The drawing under review shows one solid part. Ordinate dimensions are in mm from its lowest x, y, z. A direction names the side the tool comes from. Give positions to 0.01 mm unless a question says otherwise; leave off trailing zeros. Order: outer loops, then holes, each group sorted by start corner. A loop starts at its lowest first (then second) coordinate and runs counter-clockwise, first axis right, second up. Notation, with made-up numbers: M 17,13 L 23,13 A20 ccw 23,41 Z; hole C 35.5,55 d9. An arc over 180 degrees is marked long. Put each result on its own line as item: value. Start each with the question number.
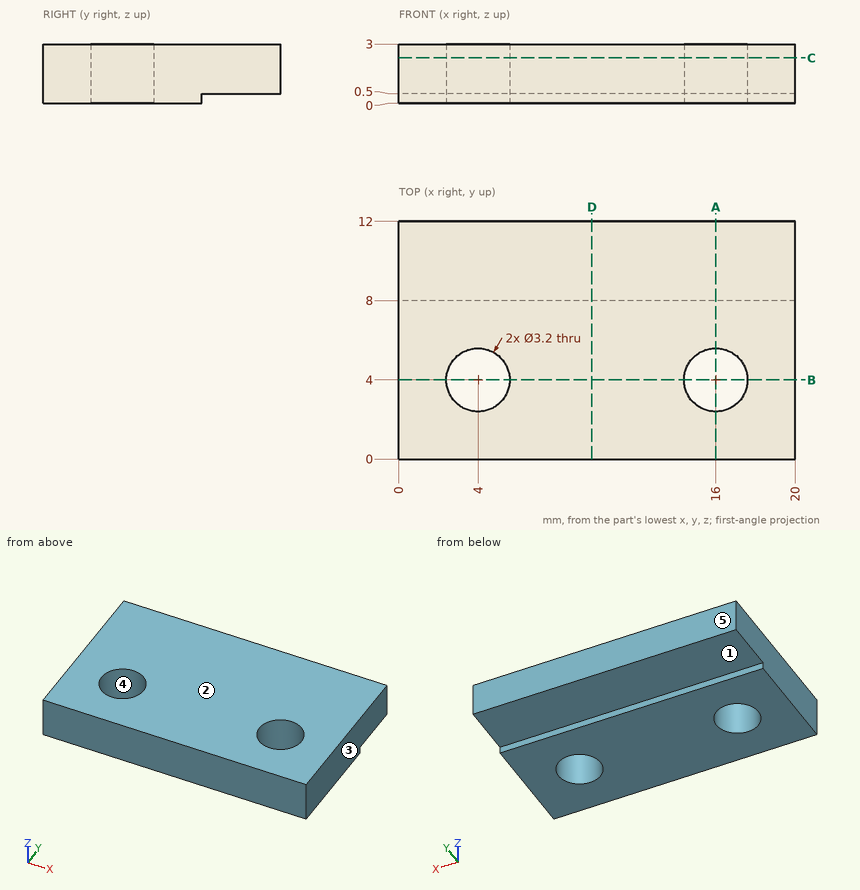
1. To check wall thickness, follow probe 1 along Y at (x, z) = (4, 1.35); probe 2 along X at (y, z) = (5.25, 1.4); probe 3 along Z at (x, y) = (18.75, 10.5). State the ranges of each line that lie inside material, in increasing order.
2. Consider section B-B on y = 4. Give the boundary of the cut face in (x, z), then the cut area to 3 significant figures.
3. Consider section C-C on z = 2.3. Give the boundary of the cut face in (x, y), then the cut area to 3 significant figures.
4. The part is to be moulded in two halves that separate along X. For the marked faces 3, 4 and 5, say which applies: +X half, -X half, draft (parallel to the pull), parting line (faces both ways), or undercut.
5. Insertion check: pin 1 (2 mm diameter, centred on x = 13, y = 10, fed in from -Z); pin 2 (3 mm diameter, centred on x = 4, y = 4, fed in from -Z). Each pin has a flat end and moves straight along its axis. Give the tip position at first contact, or say it passes through.
6. Consider section A-A on x = 16. Give the boundary of the cut face in (y, z).
7. Machinability: for the marked faces 1 and 2, which of the approach directions +Z, -Z, +X, -X, +Y, -Y give a long, thin tool a straight path to every point of the face, cutting with its end or side? Answer none if there is none.
8. Consider section D-D on x = 9.75. Give the boundary of the cut face in (y, z).
Returned:
1. probe 1: y = 0 to 2.4, 5.6 to 12
1. probe 2: x = 0 to 3, 5 to 15, 17 to 20
1. probe 3: z = 0.5 to 3
2. outline: M 0,0 L 2.4,0 L 2.4,3 L 0,3 Z; M 5.6,0 L 14.4,0 L 14.4,3 L 5.6,3 Z; M 17.6,0 L 20,0 L 20,3 L 17.6,3 Z
2. area: 40.8 mm2
3. outline: M 0,0 L 20,0 L 20,12 L 0,12 Z; hole C 4,4 d3.2; hole C 16,4 d3.2
3. area: 224 mm2
4. face 3: +X half
4. face 4: undercut
4. face 5: draft
5. pin 1: stops at z = 0.5
5. pin 2: passes through
6. outline: M 0,0 L 2.4,0 L 2.4,3 L 0,3 Z; M 5.6,0 L 8,0 L 8,0.5 L 12,0.5 L 12,3 L 5.6,3 Z
7. face 1: -Z, +X, -X, +Y
7. face 2: +Z, +X, -X, +Y, -Y
8. outline: M 0,0 L 8,0 L 8,0.5 L 12,0.5 L 12,3 L 0,3 Z
